Read the model definition and answer for the solid it produces. Units are mm, in the model's axes. Face numbers are marked on the shaded views. A direction names the side the tool comes from. Round coordinates to 2 decimals unless told otherwise and drop trailing zeros. Loops run counter-clockwise (first coordinate to the right, second up) from the corner with the lowest first, then second, coordinate; pieces in that order, holes last. Notation, with made-up numbers: (13.5, 87.25) - (37.5, 87.25) arc R29 ccw to (37.5, 125.25) - close; hole circle Ø1 at (-23, -33). An arc over 180 degrees is marked (long way). Use CSV: the item, a comma, the result in double quotes. Start each with the question number.
1. Determine the mould class of the marked faces 4, 5 and 6 for opening direction Y: +Y half, -Y half, draft (parallel to the pull), parting line (faces both ways), or undercut.
2. Find section A-A (x = -39.5). Give the vertices of the cut face in (y, z).
3. Find section C-C (x = 2.8). Give the vertices of the cut face in (y, z).
4. Find section B-B (z = 25). Give the vertices of the cut face in (x, y).
5. Find section D-D (z = 18). Give the vertices of the cut face in (x, y).
6. A tool of negligible diameter and unlimited length cuts with its end or side. For the marked faces 1, 2 and 3, from which of +Z, -Z, +X, -X, +Y, -Y can it reach the whole face along a straight path? Write none if from no direction.
7. Given pin 1 Ø1 at (x, z) = (9, -1) entering from +Y; pin 2 Ø1.6 at (y, z) = (17, 15.5) entering from -X; pin 3 Ø2 at (x, y) = (-29, -13) entering from +Z, each flat-ended and moving along its own axis, determine where each tip first touches the part or whether it passes through.
8. Consider line 1 along Y through (x, z) = (6, 18); line 2 along Z through (x, y) = (9, 9); line 3 along Z through (x, y) = (8.85, 9). Determine where each line is inside the solid, lowest interval first.
from build123d import *

# Parameters (mm, degrees)
BOSS_EXTRU_1_DEPTH        = 32
ESQUISSE2_R               = 1.55
ENL_V_MAT_EXTRU_1_DEPTH   = 39.052595181
ESQUISSE3_W               = 1.5
ESQUISSE3_H               = 7
ENL_V_MAT_EXTRU_2_DEPTH   = 39.052595181
ESQUISSE4_W               = 4
ESQUISSE4_H               = 2
BOSS_EXTRU_2_DEPTH        = 6
CONG_1_R                  = 2.5
CONG_2_R                  = 2
ESQUISSE13_R              = 2.1
ENL_V_MAT_EXTRU_3_DEPTH   = 40.293765409
ESQUISSE14_W              = 2
ESQUISSE14_H              = 14
BOSS_EXTRU_3_DEPTH        = 4
BOSS_EXTRU_4_START        = -14
ESQUISSE15_W              = 25
ESQUISSE15_H              = 2
BOSS_EXTRU_4_DEPTH        = 14
BOSS_EXTRU_5_START        = -2
BOSS_EXTRU_5_DEPTH        = 2
CONG_5_R                  = 5
CONG_6_R                  = 3
ESQUISSE26_W              = 2
ESQUISSE26_H              = 2.5
ENL_V_MAT_EXTRU_5_DEPTH   = 83.280009723
CONVERTIR_VOLUME3_DEPTH   = 32
CONVERTIR_VOLUME3_START   = 2
CONVERTIR_VOLUME3_2_DEPTH = 14
CONVERTIR_VOLUME3_3_DEPTH = 32
CONVERTIR_VOLUME3_START_2 = -6
CONVERTIR_VOLUME3_4_DEPTH = 2
CONVERTIR_VOLUME3_5_DEPTH = 14


# Read off the part's stored shape, not the designer's step: Convertir-Volume3
with BuildPart() as part:
    # Esquisse1 → Boss.-Extru.1 (new body)
    with BuildSketch(Plane.XY):
        Polygon((0, 0), (10, 0), (10, 18), (0, 18), (0, 16), (8, 16), (8, 2), (0, 2), align=None)
    extrude(amount=BOSS_EXTRU_1_DEPTH)

    # Esquisse2 → Enlèv. mat.-Extru.1 (cut, through all)
    with BuildSketch(Plane(origin=(0, 18, 0), x_dir=(1, 0, 0), z_dir=(0, 1, 0))):
        with Locations(Location((2.8, -10, 0), (0, 0, 270))):
            Circle(ESQUISSE2_R)
        with Locations((2.8, -22)):
            Circle(ESQUISSE2_R)
    extrude(amount=-ENL_V_MAT_EXTRU_1_DEPTH, mode=Mode.SUBTRACT)

    # Esquisse3 → Enlèv. mat.-Extru.2 (cut, through all)
    with BuildSketch(Plane(origin=(0, 18, 0), x_dir=(1, 0, 0), z_dir=(0, 1, 0))):
        with Locations((0.75, -16)):
            Rectangle(ESQUISSE3_W, ESQUISSE3_H)
    extrude(amount=-ENL_V_MAT_EXTRU_2_DEPTH, mode=Mode.SUBTRACT)

    # Esquisse4 → Boss.-Extru.2 (add)
    with BuildSketch(Plane.ZY):
        with Locations((2, 17)):
            Rectangle(ESQUISSE4_W, ESQUISSE4_H)
        with Locations((2, 1)):
            Rectangle(ESQUISSE4_W, ESQUISSE4_H)
        with Locations((30, 1)):
            Rectangle(ESQUISSE4_W, ESQUISSE4_H)
        with Locations((30, 17)):
            Rectangle(ESQUISSE4_W, ESQUISSE4_H)
    extrude(amount=BOSS_EXTRU_2_DEPTH)

    # Congé1
    # the kernel refuses this fillet: 2.5 mm, written as the material it takes off along each edge
    with BuildSketch(Plane(origin=(0, 7.728219619, 19.5), x_dir=(0, 0, 1), z_dir=(0, -1, 0)), Plane(origin=(0, 23.728219619, 19.5), x_dir=(0, 0, 1), z_dir=(0, -1, 0))) as cong_1_piece_1:
        with BuildLine():
            CenterArc((2.291287847, -2.5), CONG_1_R, 90, 66.421821522)
            Line((0, -1.5), (-0.045825757, -1.48))
            ThreePointArc((-0.045825757, -1.48), (-0.05, -0.75), (-0.05, 0))
            Line((-0.05, 0), (0, 0.05))
            Line((0, 0.05), (2.291287847, 0.05))
            Line((2.291287847, 0.05), (2.291287847, 0))
        make_face()
    extrude(amount=13.456439237, mode=Mode.SUBTRACT)
    with BuildSketch(Plane(origin=(0, 7.728219619, 12.5), x_dir=(1, 0, 0), z_dir=(0, -1, 0)), Plane(origin=(0, 23.728219619, 12.5), x_dir=(1, 0, 0), z_dir=(0, -1, 0))) as cong_1_piece_2:
        with BuildLine():
            CenterArc((2.5, -2.291287847), CONG_1_R, 113.578178478, 66.421821522)
            Line((0, -2.291287847), (-0.05, -2.291287847))
            Line((-0.05, -2.291287847), (-0.05, 0))
            Line((-0.05, 0), (0, 0.05))
            ThreePointArc((0, 0.05), (0.75, 0.05), (1.48, 0.045825757))
            Line((1.48, 0.045825757), (1.5, 0))
        make_face()
    extrude(amount=13.456439237, mode=Mode.SUBTRACT)

    # Congé2
    cong_2_edges = [part.edges().sort_by_distance(p)[0] for p in [
        (-6, 17, 32),
        (-6, 17, 0),
        (-6, 1, 0),
        (-6, 1, 32),
    ]]
    fillet(cong_2_edges, radius=CONG_2_R)

    # Esquisse13 → Enlèv. mat.-Extru.3 (cut, through all)
    with BuildSketch(Plane.ZY.offset(-8)):
        with Locations(Location((7, 9, 0), (0, 0, 270))):
            Circle(ESQUISSE13_R)
        with Locations(Location((25, 9, 0), (0, 0, 90))):
            Circle(ESQUISSE13_R)
    extrude(amount=-ENL_V_MAT_EXTRU_3_DEPTH, mode=Mode.SUBTRACT)

    # Esquisse14 → Boss.-Extru.3 (add)
    with BuildSketch(Plane(origin=(0, 0, 0), x_dir=(-1, 0, 0), z_dir=(0, 0, -1))):
        with Locations((-9, 9)):
            Rectangle(ESQUISSE14_W, ESQUISSE14_H)
    extrude(amount=BOSS_EXTRU_3_DEPTH)

    # Esquisse15 → Boss.-Extru.4 (add)
    with BuildSketch(Plane.XZ.offset(-2).offset(BOSS_EXTRU_4_START)):
        with Locations((-2.5, -5)):
            Rectangle(ESQUISSE15_W, ESQUISSE15_H)
    extrude(amount=BOSS_EXTRU_4_DEPTH)

    # Esquisse16 → Boss.-Extru.5 (add)
    with BuildSketch(Plane(origin=(0, 0, -6), x_dir=(-1, 0, 0), z_dir=(0, 0, -1)).offset(BOSS_EXTRU_5_START)):
        Polygon((15, 16), (15, 39), (55, 39), (55, 22.5), (30, 22.5), (30, -4.5), (55, -4.5), (55, -21), (15, -21), (15, 2), align=None)
    extrude(amount=BOSS_EXTRU_5_DEPTH)

    # Congé5
    cong_5_edges = [part.edges().sort_by_distance(p)[0] for p in [
        (-15, 16, -5),
        (-15, 2, -5),
        (-15, -21, -5),
        (-15, 39, -5),
        (-55, 39, -5),
        (-55, 22.5, -5),
        (-55, -4.5, -5),
        (-55, -21, -5),
    ]]
    fillet(cong_5_edges, radius=CONG_5_R)

    # Congé6
    cong_6_edges = [part.edges().sort_by_distance(p)[0] for p in [
        (-30, 22.5, -5),
        (-30, -4.5, -5),
    ]]
    fillet(cong_6_edges, radius=CONG_6_R)

    # Esquisse26 → Enlèv. mat.-Extru.5 (cut, through all)
    with BuildSketch(Plane(origin=(10, 0, 0), x_dir=(0, 0, -1), z_dir=(1, 0, 0))):
        with Locations((1, 3.25)):
            Rectangle(ESQUISSE26_W, ESQUISSE26_H)
        with Locations((1, 14.75)):
            Rectangle(ESQUISSE26_W, ESQUISSE26_H)
    extrude(amount=-ENL_V_MAT_EXTRU_5_DEPTH, mode=Mode.SUBTRACT)

    # Convertir-Volume3 outline → Convertir-Volume3 (add)
    with BuildSketch(Plane.XY):
        with BuildLine():
            ThreePointArc((6, 16), (7.414213562, 15.414213562), (8, 14))
            Line((8, 14), (8, 16))
            Line((8, 16), (6, 16))
        make_face()
        with BuildLine():
            Line((8, 2), (8, 4))
            ThreePointArc((8, 4), (7.414213562, 2.585786438), (6, 2))
            Line((6, 2), (8, 2))
        make_face()
    extrude(amount=CONVERTIR_VOLUME3_DEPTH)

    # Convertir-Volume3 2 outline → Convertir-Volume3 2 (add)
    with BuildSketch(Plane(origin=(0, 0, 0), x_dir=(1, 0, 0), z_dir=(0, 1, 0)).offset(CONVERTIR_VOLUME3_START)):
        with BuildLine():
            ThreePointArc((6, 4), (7.414213562, 3.414213562), (8, 2))
            Line((8, 2), (8, 4))
            Line((8, 4), (6, 4))
        make_face()
    extrude(amount=CONVERTIR_VOLUME3_2_DEPTH)

    # Convertir-Volume3 3 outline → Convertir-Volume3 3 (cut)
    with BuildSketch(Plane.XY):
        with BuildLine():
            Line((10, 14), (10, 18))
            Line((10, 18), (6, 18))
            ThreePointArc((6, 18), (8.828427125, 16.828427125), (10, 14))
        make_face()
        with BuildLine():
            Line((10, 0), (10, 4))
            ThreePointArc((10, 4), (8.828427125, 1.171572875), (6, 0))
            Line((6, 0), (10, 0))
        make_face()
    extrude(amount=CONVERTIR_VOLUME3_3_DEPTH, mode=Mode.SUBTRACT)

    # Convertir-Volume3 4 outline → Convertir-Volume3 4 (cut)
    with BuildSketch(Plane.XY.offset(CONVERTIR_VOLUME3_START_2)):
        with BuildLine():
            Line((10, 16), (9.464101616, 16))
            ThreePointArc((9.464101616, 16), (9.863703305, 15.03527618), (10, 14))
            Line((10, 14), (10, 16))
        make_face()
        with BuildLine():
            ThreePointArc((10, 4), (9.863703305, 2.96472382), (9.464101616, 2))
            Line((9.464101616, 2), (10, 2))
            Line((10, 2), (10, 4))
        make_face()
    extrude(amount=CONVERTIR_VOLUME3_4_DEPTH, mode=Mode.SUBTRACT)

    # Convertir-Volume3 5 outline → Convertir-Volume3 5 (cut)
    with BuildSketch(Plane(origin=(0, 0, 0), x_dir=(1, 0, 0), z_dir=(0, 1, 0)).offset(CONVERTIR_VOLUME3_START)):
        with BuildLine():
            ThreePointArc((6, 6), (8.828427125, 4.828427125), (10, 2))
            Line((10, 2), (10, 6))
            Line((10, 6), (6, 6))
        make_face()
    extrude(amount=CONVERTIR_VOLUME3_5_DEPTH, mode=Mode.SUBTRACT)


solid = part.part
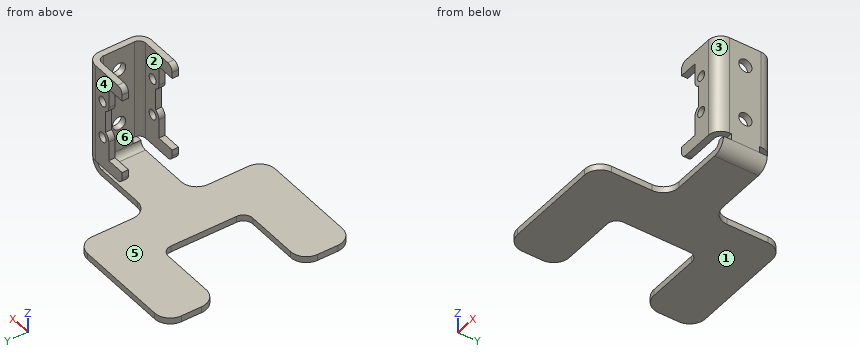
Filled sheet:
1,face 4,"+Y half"
1,face 5,"draft"
1,face 6,"undercut"
2,outline,"(-21, -6) - (-4.5, -6) - (-4.5, -4) - (-21, -4) - close; (22.5, -6) - (39, -6) - (39, -4) - (22.5, -4) - close"
3,outline,"(0, 0) - (2, 0) - (2, 8.45) - (0, 8.45) - close; (0, 11.55) - (2, 11.55) - (2, 20.45) - (0, 20.45) - close; (0, 23.55) - (2, 23.55) - (2, 32) - (0, 32) - close; (2, -6) - (16, -6) - (16, -4) - (2, -4) - close; (16, 0) - (18, 0) - (18, 8.45) - (16, 8.45) - close; (16, 11.55) - (18, 11.55) - (18, 20.45) - (16, 20.45) - close; (16, 23.55) - (18, 23.55) - (18, 32) - (16, 32) - close"
4,outline,"(0, 0) - (6, 0) arc R4 ccw to (10, 4) - (10, 6.9) - (8, 6.9) - (8, 4) arc R2 cw to (6, 2) - (0, 2) - close; (0, 16) - (6, 16) arc R2 cw to (8, 14) - (8, 11.1) - (10, 11.1) - (10, 14) arc R4 ccw to (6, 18) - (0, 18) - close"
5,outline,"(1.5, 0) - (6, 0) arc R4 ccw to (10, 4) - (10, 14) arc R4 ccw to (6, 18) - (1.5, 18) - (1.5, 16) - (6, 16) arc R2 cw to (8, 14) - (8, 4) arc R2 cw to (6, 2) - (1.5, 2) - close"
6,face 1,"-Z, +X, -X, +Y, -Y"
6,face 2,"+Z, -X"
6,face 3,"+Z, +X, -Y"
7,pin 1,"stops at y = 13.5"
7,pin 2,"stops at x = 1.5"
7,pin 3,"stops at z = -4"
8,line 1,"y = 0 to 2, 16 to 18"
8,line 2,"z = -4.65 to 4.9, 9.1 to 22.9, 27.1 to 32"
8,line 3,"z = -4.81 to 4.9, 9.1 to 22.9, 27.1 to 32"
